Could you check a few things on this model? Use its own coordinates, in mm. A direction names the side the tool comes from. Round coordinates to 2 decimals unless told otherwise and drop trailing zeros. Order: outer loops, then holes, each group sorted by start corner. A loop starts at its lowest first (then second) coordinate and runs counter-clockwise, first axis right, second up. Notation, with made-up numbers: (-34, -14) -> (13, -14) arc R22 cw to (13, 11) -> close; hole circle Ø4 at (8.5, 41.5). An arc over 180 degrees is marked (long way). One line per question, with ' | ' between items.
Autodesk Inventor part; units mm, degrees
ref_plane "YZ Plane" through (0, 0, 0) normal (1, 0, 0) x (0, 1, 0)
ref_plane "XZ Plane" through (0, 0, 0) normal (0, 1, 0) x (-1, 0, 0)
ref_plane "XY Plane" through (0, 0, 0) normal (0, 0, 1) x (1, 0, 0)
sketch "スケッチ1" plane through (0, 0, 0) normal (0, 1, 0) x (-1, 0, 0)
  line L0 (0, 0) -> (0, 25)
  line L1 (0, 25) -> (0, 104.965)
  line L2 (0, 104.965) -> (0, 139.606)
  line L3 (-45, 25) -> (45, 25)
  line L4 (45, 25) -> (45, 0)
  line L5 (45, 0) -> (-45, 0)
  line L6 (-45, 0) -> (-45, 25)
  line L7 (-45, 25) -> (45, 0) construction
  line L8 (45, 25) -> (-45, 0) construction
  line L9 (-47, 28) -> (47, 28)
  line L10 (47, 28) -> (47, -3)
  line L11 (47, -3) -> (-47, -3)
  line L12 (-47, -3) -> (-47, 28)
  line L13 (-47, 28) -> (47, -3) construction
  line L14 (47, 28) -> (-47, -3) construction
  line L15 (-47, 142.2855) -> (47, 142.2855)
  line L16 (47, 142.2855) -> (47, 102.2855)
  line L17 (47, 102.2855) -> (-47, 102.2855)
  line L18 (-47, 102.2855) -> (-47, 142.2855)
  line L19 (-47, 142.2855) -> (47, 102.2855) construction
  line L20 (47, 142.2855) -> (-47, 102.2855) construction
  line L21 (-45, 139.606) -> (45, 139.606)
  line L22 (45, 139.606) -> (45, 104.965)
  line L23 (45, 104.965) -> (-45, 104.965)
  line L24 (-45, 104.965) -> (-45, 139.606)
  line L25 (-45, 139.606) -> (45, 104.965) construction
  line L26 (45, 139.606) -> (-45, 104.965) construction
  line L27 (-10, 28) -> (10, 28)
  line L28 (10, 28) -> (10, 102.2855)
  line L29 (10, 102.2855) -> (-10, 102.2855)
  line L30 (-10, 102.2855) -> (-10, 28)
  arc A0 (-10, 84.5837) -> (-47, 102.2855) centre (-46.0082, 56.8392) ccw
  arc A1 (-47, 28) -> (-10, 49.4601) centre (-44.5907, 66.4724) ccw
  arc A2 (47, 102.2855) -> (10, 84.5837) centre (46.0082, 56.8392) ccw
  arc A3 (10, 49.4601) -> (47, 28) centre (44.5907, 66.4724) ccw
  point P0 (0, 12.5)
  point P1 (0, 12.5)
  point P2 (0, 122.2855)
  point P3 (0, 122.2855)
  dimension "d0" = 25
  dimension "d1" = 79.965
  dimension "d2" = 34.641
  dimension "d3" = 90
  dimension "d4" = 94
  dimension "d5" = 31
  dimension "d6" = 94
  dimension "d7" = 40
  dimension "d8" = 90
  dimension "d9" = 20
  dimension "d10" = 10
extrude "押し出し1" add sketch "スケッチ1" along normal blind 3 contours L9 L30 L17 L1 | L9 A3 L10 L11 L12 A1 | L1 L17 L28 L9 | L17 A0 L18 L15 L16 A2 | A1 L9 | L9 A3 | A2 L17 | L17 A0
sketch "スケッチ2" plane through (0, 3, 0) normal (0, 1, 0) x (1, 0, 0)
  line L0 (-45, -139.606) -> (-45, -104.965)
  line L1 (-45, -104.965) -> (45, -104.965)
  line L2 (45, -104.965) -> (45, -139.606)
  line L3 (45, -139.606) -> (-45, -139.606)
  line L4 (-45, -25) -> (-45, 0)
  line L5 (-45, 0) -> (45, 0)
  line L6 (45, 0) -> (45, -25)
  line L7 (45, -25) -> (-45, -25)
  line L8 (-10, -28) -> (-10, -102.2855)
  line L9 (-10, -102.2855) -> (-47, -102.2855)
  line L10 (-47, -102.2855) -> (-47, -142.2855)
  line L11 (-47, -142.2855) -> (47, -142.2855)
  line L12 (47, -142.2855) -> (47, -102.2855)
  line L13 (47, -102.2855) -> (10, -102.2855)
  line L14 (10, -102.2855) -> (10, -28)
  line L15 (10, -28) -> (47, -28)
  line L16 (47, -28) -> (47, 3)
  line L17 (47, 3) -> (-47, 3)
  line L18 (-47, 3) -> (-47, -28)
  line L19 (-47, -28) -> (-10, -28)
  arc A0 (-10, -47.2222) -> (-47, -28) centre (-44.6937, -68.7817) ccw
  arc A1 (-47, -102.2855) -> (-10, -81.2921) centre (-44.5262, -63.5433) ccw
  line L20 (0, -57.408) -> (0, -62.3253)
  arc A2 (47, -28) -> (10, -47.2222) centre (44.6937, -68.7817) ccw
  arc A3 (10, -81.2921) -> (47, -102.2855) centre (44.5262, -63.5433) ccw
  arc A4 (-10, -47.2222) -> (-47, -28) centre (-44.6937, -68.7817) ccw
  arc A5 (-47, -102.2855) -> (-10, -81.2921) centre (-44.5262, -63.5433) ccw
  arc A6 (47, -28) -> (10, -47.2222) centre (44.6937, -68.7817) ccw
  arc A7 (10, -81.2921) -> (47, -102.2855) centre (44.5262, -63.5433) ccw
  point P0 (0, 0)
sketch "スケッチ3" plane through (0, 3, 0) normal (0, 1, 0) x (1, 0, 0)
  line L0 (-45, -139.606) -> (-45, -104.965)
  line L1 (-45, -104.965) -> (45, -104.965)
  line L2 (45, -104.965) -> (45, -139.606)
  line L3 (45, -139.606) -> (-45, -139.606)
  line L4 (-45, -25) -> (-45, 0)
  line L5 (-45, 0) -> (45, 0)
  line L6 (45, 0) -> (45, -25)
  line L7 (45, -25) -> (-45, -25)
  line L8 (-10, -28) -> (-10, -102.2855)
  line L9 (-10, -102.2855) -> (-47, -102.2855)
  line L10 (-47, -102.2855) -> (-47, -142.2855)
  line L11 (-47, -142.2855) -> (47, -142.2855)
  line L12 (47, -142.2855) -> (47, -102.2855)
  line L13 (47, -102.2855) -> (10, -102.2855)
  line L14 (10, -102.2855) -> (10, -28)
  line L15 (10, -28) -> (47, -28)
  line L16 (47, -28) -> (47, 3)
  line L17 (47, 3) -> (-47, 3)
  line L18 (-47, 3) -> (-47, -28)
  line L19 (-47, -28) -> (-10, -28)
  arc A0 (-10, -47.2222) -> (-47, -28) centre (-44.6589, -68.7147) ccw
  arc A1 (47, -28) -> (10, -47.2222) centre (45.0843, -69.5335) ccw
  arc A2 (10, -81.5262) -> (47, -102.2855) centre (44.8559, -62.7542) ccw
  arc A3 (-47, -102.2855) -> (-10, -81.5262) centre (-44.3224, -63.705) ccw
  point P0 (0, 0)
extrude "押し出し3" add sketch "スケッチ3" against normal blind 3 contours L19 A0 L18 L17 L16 A1 L15 L14 L13 A2 L12 L11 L10 A3 L9 L8 | L8 A0 L19 | L19 A0 | L8 L9 A3 | A3 L9 | L15 A1 | A2 L13
sketch "スケッチ4" plane through (0, 3, 0) normal (0, 1, 0) x (1, 0, 0)
  line L0 (-45, -139.606) -> (-45, -104.965)
  line L1 (-45, -104.965) -> (45, -104.965)
  line L2 (45, -104.965) -> (45, -139.606)
  line L3 (45, -139.606) -> (-45, -139.606)
  line L4 (-45, -25) -> (-45, 0)
  line L5 (-45, 0) -> (45, 0)
  line L6 (45, 0) -> (45, -25)
  line L7 (45, -25) -> (-45, -25)
  line L8 (-10, -47.2222) -> (-10, -81.5262)
  arc A0 (-41.6448, -102.2855) -> (-10, -81.5262) centre (-44.3224, -63.705) ccw
  line L9 (-41.6448, -102.2855) -> (-47, -102.2855)
  line L10 (-47, -102.2855) -> (-47, -142.2855)
  line L11 (-47, -142.2855) -> (47, -142.2855)
  line L12 (47, -142.2855) -> (47, -102.2855)
  line L13 (47, -102.2855) -> (10, -102.2855)
  line L14 (10, -102.2855) -> (10, -28)
  line L15 (10, -28) -> (47, -28)
  line L16 (47, -28) -> (47, 3)
  line L17 (47, 3) -> (-47, 3)
  line L18 (-47, 3) -> (-47, -28)
  line L19 (-47, -28) -> (-42.3178, -28)
  arc A1 (-10, -47.2222) -> (-42.3178, -28) centre (-44.6589, -68.7147) ccw
  arc A2 (47, -28) -> (10, -47.2222) centre (45.7708, -70.8549) ccw
  arc A3 (10, -81.5262) -> (47, -102.2855) centre (45.1409, -62.2461) ccw
  point P0 (0, 0)
extrude "押し出し4" add sketch "スケッチ4" against normal blind 3
sketch "スケッチ5" plane through (0, 0, 0) normal (0, -1, 0) x (1, 0, 0)
  arc A0 (43.2819, 102.2855) -> (10, 81.5262) centre (45.1409, 62.2461) ccw
  line L0 (47, 102.2855) -> (43.2819, 102.2855)
  line L1 (47, 142.2855) -> (47, 102.2855)
  line L2 (-47, 142.2855) -> (47, 142.2855)
  line L3 (-47, 102.2855) -> (-47, 142.2855)
  line L4 (-41.6448, 102.2855) -> (-47, 102.2855)
  arc A1 (-10, 81.5262) -> (-41.6448, 102.2855) centre (-44.3224, 63.705) ccw
  line L5 (-10, 47.2222) -> (-10, 81.5262)
  arc A2 (-42.3178, 28) -> (-10, 47.2222) centre (-44.6589, 68.7147) ccw
  line L6 (-47, 28) -> (-42.3178, 28)
  line L7 (-47, -3) -> (-47, 28)
  line L8 (47, -3) -> (-47, -3)
  line L9 (47, 28) -> (47, -3)
  line L10 (44.5416, 28) -> (47, 28)
  arc A3 (10, 47.2222) -> (44.5416, 28) centre (45.7708, 70.8549) ccw
  line L11 (10, 81.5262) -> (10, 47.2222)
  point P0 (0, 0)
extrude "押し出し5" add sketch "スケッチ5" along normal blind 2
sketch "スケッチ6" plane through (0, 3, 0) normal (0, 1, 0) x (1, 0, 0)
  line L0 (45, -104.965) -> (-45, -104.965)
  line L1 (-45, -104.965) -> (-45, -104.865)
  line L2 (-45, -104.865) -> (45, -104.865)
  line L3 (45, -104.865) -> (45, -104.965)
  point P0 (0, 0)
  dimension "d21" = 0.1
extrude "押し出し6" cut sketch "スケッチ6" against normal blind 3
sketch "スケッチ7" plane through (-10, 3, 47.2222) normal (-1, 0, 0) x (0, 0, 1)
  line L0 (34.3041, -5) -> (0, -5)
  line L1 (57.6402, 0) -> (44.0812, 0)
  line L2 (44.0812, 0) -> (54.2504, 5.8712)
  line L3 (57.6402, 0) -> (54.2504, 5.8712)
  point P0 (-47.2222, -3)
  dimension "d24" = 30
extrude "押し出し7" add sketch "スケッチ7" against normal blind 20
sketch "スケッチ8" plane through (-10, 3, 47.2222) normal (-1, 0, 0) x (0, 0, 1)
  line L0 (57.6402, 0) -> (44.0812, 0)
  line L1 (54.2504, 5.8712) -> (57.6402, 0)
  line L2 (44.0812, 0) -> (54.2504, 5.8712)
  line L3 (57.6402, 0) -> (48.1987, 16.3532)
  line L4 (44.0812, 13.9759) -> (44.0812, 0)
  line L5 (44.0812, 13.9759) -> (48.1987, 16.3532)
  point P0 (-47.2222, -3)
  dimension "d27" = 18.883
extrude "押し出し8" add sketch "スケッチ8" against normal blind 20 contours L4 L5 L3 L2
sketch "スケッチ9" plane through (-10, 3, 47.2222) normal (-1, 0, 0) x (0, 0, 1)
  line L0 (48.1987, 16.3532) -> (44.0812, 13.9759)
  line L1 (44.0812, 13.9759) -> (44.0812, 0)
  line L2 (48.1987, 16.3532) -> (47.6747, 17.2608)
  line L3 (47.6747, 17.2608) -> (43.5572, 14.8835)
  line L4 (43.5572, 14.8835) -> (44.0812, 13.9759)
  line L5 (44.0812, 13.9759) -> (48.1987, 16.3532)
  line L6 (44.0812, 13.9759) -> (44.0812, 15.1861)
  point P0 (-47.2222, -3)
  dimension "d30" = 1.048
extrude "押し出し9" add sketch "スケッチ9" against normal blind 20 contours L0 L6 L3 L2
sketch "スケッチ10" plane through (-10, 3, 47.2222) normal (-1, 0, 0) x (0, 0, 1)
  line L0 (57.6402, 0) -> (44.0812, 0)
  line L1 (57.6402, 0) -> (47.6747, 17.2608)
  line L2 (47.6747, 17.2608) -> (44.0812, 15.1861)
  line L3 (44.0812, 15.1861) -> (44.0812, 0)
  point P0 (-47.2222, -3)
extrude "押し出し10" cut sketch "スケッチ10" against normal blind 20
sketch "スケッチ11" plane through (0, -2, 0) normal (0, -1, 0) x (1, 0, 0)
  line L0 (-47, -3) -> (47, -3)
  line L1 (10, 47.2222) -> (10, 81.5262)
  line L2 (0, -3) -> (0, 47)
  line L3 (0, 47) -> (0, 57)
  line L4 (0, 57) -> (0, 67)
  line L5 (0, 67) -> (0, 77)
  line L6 (0, 77) -> (0, 87)
  circle A0 centre (0, 47) radius 1.5
  circle A1 centre (0, 57) radius 1.5
  circle A2 centre (0, 67) radius 1.5
  circle A3 centre (0, 77) radius 1.5
  circle A4 centre (0, 87) radius 1.5
  point P0 (0, 0)
  dimension "d35" = 50
  dimension "d36" = 10
  dimension "d37" = 10
  dimension "d38" = 10
  dimension "d39" = 10
  dimension "d40" = 3
  dimension "d41" = 3
  dimension "d42" = 3
  dimension "d43" = 3
  dimension "d44" = 3
hole "穴1" at (0, -2, 87) at (0, -2, 77) at (0, -2, 67) at (0, -2, 57) at (0, -2, 47) direction (0, 1, 0) diameter 3 depth 8 tip angle 118
properties part number "知能ロボコン台座" material "ABS プラスチック"
1. I need wall thicknesses on probe 1 along X at (y, z) = (0.3, 136); probe 2 along Z at (x, y) = (2.5, 1.75) (1 decimal); probe 3 along X at (y, z) = (1.8, 57). Which ranges of each line are inside material? Lowest first, please.
From the geometry:
probe 1: x = -47 to -45, 45 to 47 | probe 2: z = -3 to 0, 25 to 104.9, 139.6 to 142.3 | probe 3: x = -10 to -1.5, 1.5 to 10
2. If we mould it in two halves opening along X, with no side actions, what happens to faces 4 (the face through (45, 1, 102.286)), 5 (the face through (-0.45, 0.54, 55.57)), 6 (the face through (-23.34, 1.52, 96.19)), 7 (the face through (25.175, -0.986, 33.253))? For each: pulls with the +X half, pulls with the -X half, needs draft (parallel to the pull), parting line crosses it, or undercut.
From the geometry:
face 4: needs draft | face 5: undercut | face 6: pulls with the -X half | face 7: pulls with the +X half
3. I want a section at A-A on z = 77. List the corners of the cut face in (x, y) for me.
From the geometry:
outline: (-10, -2) -> (-1.5, -2) -> (-1.5, 3) -> (-10, 3) -> close; (1.5, -2) -> (10, -2) -> (10, 3) -> (1.5, 3) -> close
4. I'm going to push flat-ended pins straight in: pin 1 (2.5 mm diameter, centred on y = 1.5, z = 68.5, fed in from -X); pin 2 (2.5 mm diameter, centred on y = 0.5, z = 71.5, fed in from +X); pin 3 (1.5 mm diameter, centred on y = 1, z = 36.5, fed in from -X). Where does each tip first touch, or does it pass through?
From the geometry:
pin 1: stops at x = -10 | pin 2: stops at x = 10 | pin 3: stops at x = -20.65
5. I want a section at B-B on x = 0. Count the separate pieces of the cut face and the enclosed holes in it, and give its area (3 significant figures).
From the geometry:
separate pieces: 6 | enclosed holes: 0 | area: 472 mm²
6. On a 3-axis mill with a long thin cutter (end or side, diameter ignored), from which of +Z, -Z, +X, -X, +Y, -Y can I reach the whole of each face in a straight line? I mean faces 1 (the face through (1, 1, 25)), 2 (the face through (-23.34, -0.99, 96.19)), 3 (the face through (23.685, 1.521, 96.103)). Say none if no direction works.
From the geometry:
face 1: +Y | face 2: -X, +Y, -Y | face 3: +X, +Y, -Y
7. I want a section at D-D on z = 8.5. List the corners of the cut face in (x, y) for me.
From the geometry:
outline: (-47, -2) -> (47, -2) -> (47, 3) -> (45, 3) -> (45, 0) -> (-45, 0) -> (-45, 3) -> (-47, 3) -> close
